Check sheet for the drawn part. Datum: minimum x, y, z corner. Units: mm. Give positions to 0.01 mm unless a question says otherwise; leave off trailing zeros. Order: outer loops, then holes, each group sorted by start corner. A loop starts at its lowest first (then second) coordinate and runs counter-clockwise, first axis right, second up.
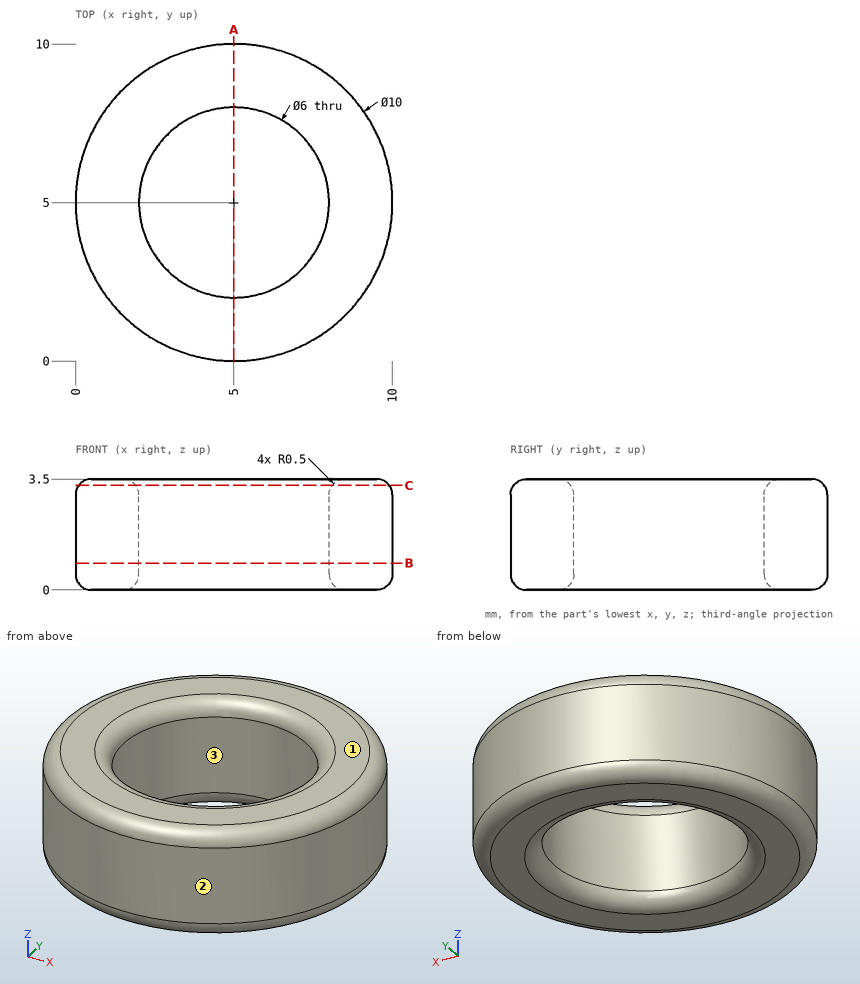
Q1. Material ranges on line 1 (Y direction, x = 5, z = 2.35); line 2 (Y direction, x = 3, z = 2.15); line 3 (Y direction, x = 9, z = 0.55), recorded low to high.
Q2. Sectioned sample at A-A, the plane x = 5. Record the cut outline in (y, z).
Q3. Sectioned sample at C-C, the plane z = 3.3. Record the cut outline in (x, y), plus the area to 3 significant figures.
Q4. Draft check along X on the marked faces 1, 2 and 3. Enter one of: pulls with the +X half, pulls with the -X half, needs draft (parallel to the pull), parting line crosses it, or undercut.
Q5. Sectioned sample at B-B, the plane z = 0.85. Record the cut outline in (x, y), plus the area to 3 significant figures.
Q6. Go/stop test with flat-tipped pins: P1, Ø1.5, axis at y = 8, z = 2.5, coming from the -X side; P2, Ø2, axis at x = 9, z = 0.5, coming from the +Y side; P3, Ø1.5, axis at y = 6, z = 1, coming from the -X side. Record where each tip stops, or that it passes through.
Filled in:
1. line 1: y = 0 to 2, 8 to 10
1. line 2: y = 0.42 to 2.76, 7.24 to 9.58
1. line 3: y = 2 to 8
2. outline: (0, 0.5) arc R0.5 ccw to (0.5, 0) - (1.5, 0) arc R0.5 ccw to (2, 0.5) - (2, 3) arc R0.5 ccw to (1.5, 3.5) - (0.5, 3.5) arc R0.5 ccw to (0, 3) - close; (8, 0.5) arc R0.5 ccw to (8.5, 0) - (9.5, 0) arc R0.5 ccw to (10, 0.5) - (10, 3) arc R0.5 ccw to (9.5, 3.5) - (8.5, 3.5) arc R0.5 ccw to (8, 3) - close
3. outline: circle Ø9.8 at (5, 5); hole circle Ø6.2 at (5, 5)
3. area: 45.2 mm2
4. face 1: needs draft
4. face 2: parting line crosses it
4. face 3: undercut
5. outline: circle Ø10 at (5, 5); hole circle Ø6 at (5, 5)
5. area: 50.3 mm2
6. P1: stops at x = 0.53
6. P2: stops at y = 9
6. P3: stops at x = 0.01
